```python
from build123d import *

# Parameters (mm, degrees)
SKETCH1_R           = 1.25
BOSS_EXTRUDE1_DEPTH = 3
SKETCH8_R           = 2.45
SKETCH8_R_2         = 1.85
CUT_EXTRUDE3_DEPTH  = 0.8
CHAMFER4_SIZE       = 0.3
SKETCH9_R           = 3.1
CUT_EXTRUDE4_DEPTH  = 20.810156141
BOSS_EXTRUDE2_DEPTH = 14
CUT_EXTRUDE5_REACH  = 27.931
SKETCH11_W          = 1.3
SKETCH11_H          = 2.4
FILLET1_SIZE        = 0.7
FILLET1_SIZE_2      = 1.8
CUT_EXTRUDE6_REACH  = 26.043


# Some blends are built 0.0001 mm under size
with BuildPart() as part:
    # Sketch1 → Boss-Extrude1 (new body)
    with BuildSketch(Plane(origin=(0, 0, 0), x_dir=(1, 0, 0), z_dir=(0, 1, 0))):
        with BuildLine():
            ThreePointArc((4.470296705, 10.516185401), (0, 14.5), (-4.470296705, 10.516185401))
            ThreePointArc((-4.470296705, 10.516185401), (-6.673163323, 3.852752641), (-11.342432061, -1.386702192))
            ThreePointArc((-11.342432061, -1.386702192), (-12.557368355, -7.25), (-6.872135356, -9.12948321))
            ThreePointArc((-6.872135356, -9.12948321), (0, -7.705505282), (6.872135356, -9.12948321))
            ThreePointArc((6.872135356, -9.12948321), (12.557368355, -7.25), (11.342432061, -1.386702192))
            ThreePointArc((11.342432061, -1.386702192), (6.673163323, 3.852752641), (4.470296705, 10.516185401))
        make_face()
        with Locations(Location((0, 10, 0), (0, 0, 270))):
            Circle(SKETCH1_R, mode=Mode.SUBTRACT)
        with Locations(Location((-8.660254038, -5, 0), (0, 0, 270))):
            Circle(SKETCH1_R, mode=Mode.SUBTRACT)
        with Locations(Location((8.660254038, -5, 0), (0, 0, 270))):
            Circle(SKETCH1_R, mode=Mode.SUBTRACT)
    extrude(amount=BOSS_EXTRUDE1_DEPTH)

    # Sketch8 → Cut-Extrude3 (cut)
    # profile 1 of 3: a face of its own
    with BuildSketch(Plane.XZ):
        with Locations(Location((8.660254038, 5, 0), (0, 0, 270))):
            Circle(SKETCH8_R)
        with Locations(Location((8.660254038, 5, 0), (0, 0, 270))):
            Circle(SKETCH8_R_2, mode=Mode.SUBTRACT)
    # profile 2 of 3: a face of its own
    with BuildSketch(Plane.XZ):
        with Locations(Location((-8.660254038, 5, 0), (0, 0, 270))):
            Circle(SKETCH8_R)
        with Locations(Location((-8.660254038, 5, 0), (0, 0, 270))):
            Circle(SKETCH8_R_2, mode=Mode.SUBTRACT)
    # profile 3 of 3: a face of its own
    with BuildSketch(Plane.XZ):
        with Locations(Location((0, -10, 0), (0, 0, 270))):
            Circle(SKETCH8_R)
        with Locations(Location((0, -10, 0), (0, 0, 270))):
            Circle(SKETCH8_R_2, mode=Mode.SUBTRACT)
    extrude(amount=-CUT_EXTRUDE3_DEPTH, mode=Mode.SUBTRACT)

    # Chamfer4
    chamfer4_edges = [part.edges().sort_by_distance(p)[0] for p in [
        (8.660254038, 0.8, 7.45),
        (8.660254038, 0.8, 6.85),
        (-8.660254038, 0.8, 7.45),
        (-8.660254038, 0.8, 6.85),
        (0, 0.8, -7.55),
        (0, 0.8, -8.15),
        (0, 0, -7.55),
    ]]
    chamfer(chamfer4_edges, length=CHAMFER4_SIZE - 0.0001)  # a hair under: the kernel refuses the full size

    # Sketch9 → Cut-Extrude4 (cut, through all)
    with BuildSketch(Plane(origin=(0, 3, 0), x_dir=(1, 0, 0), z_dir=(0, 1, 0))):
        with Locations(Location((0, 0, 0), (0, 0, 270))):
            Circle(SKETCH9_R)
    extrude(amount=-CUT_EXTRUDE4_DEPTH, mode=Mode.SUBTRACT)

    # Sketch10 → Boss-Extrude2 (add)
    with BuildSketch(Plane(origin=(0, 3, 0), x_dir=(1, 0, 0), z_dir=(0, 1, 0))):
        with BuildLine():
            ThreePointArc((-1.25, 7.603440777), (-7.705505282, 0), (-1.25, -7.603440777))
            Line((-1.25, -7.603440777), (-1.25, -5.458708638))
            ThreePointArc((-1.25, -5.458708638), (-5.6, 0), (-1.25, 5.458708638))
            Line((-1.25, 5.458708638), (-1.25, 7.603440777))
        make_face()
        with BuildLine():
            Line((1.25, -5.458708638), (1.25, -7.603440777))
            ThreePointArc((1.25, -7.603440777), (5.873954939, -4.987129939), (7.705505282, 0))
            ThreePointArc((7.705505282, 0), (5.873954939, 4.987129939), (1.25, 7.603440777))
            Line((1.25, 7.603440777), (1.25, 5.458708638))
            ThreePointArc((1.25, 5.458708638), (4.379497688, 3.489985673), (5.6, 0))
            ThreePointArc((5.6, 0), (4.379497688, -3.489985673), (1.25, -5.458708638))
        make_face()
    extrude(amount=BOSS_EXTRUDE2_DEPTH)

    # Sketch11 → Cut-Extrude5 (cut, up to next)
    with BuildSketch(Plane.XZ, mode=Mode.PRIVATE) as cut_extrude5_sk1:
        Polygon((13.271598839, 8.412916512), (11.19313787, 7.212916512), (11.84313787, 6.087083488), (13.921598839, 7.287083488), align=None)
    cut_extrude5_tool1 = extrude(cut_extrude5_sk1.sketch, amount=-CUT_EXTRUDE5_REACH, mode=Mode.PRIVATE) & part.part
    # Sketch11 → Cut-Extrude5 (cut, up to next)
    with BuildSketch(Plane.XZ, mode=Mode.PRIVATE) as cut_extrude5_sk2:
        Polygon((-13.921598839, 7.287083488), (-11.84313787, 6.087083488), (-11.19313787, 7.212916512), (-13.271598839, 8.412916512), align=None)
    cut_extrude5_tool2 = extrude(cut_extrude5_sk2.sketch, amount=-CUT_EXTRUDE5_REACH, mode=Mode.PRIVATE) & part.part
    # Sketch11 → Cut-Extrude5 (cut, up to next)
    with BuildSketch(Plane.XZ, mode=Mode.PRIVATE) as cut_extrude5_sk3:
        with Locations((0, -14.5)):
            Rectangle(SKETCH11_W, SKETCH11_H)
    cut_extrude5_tool3 = extrude(cut_extrude5_sk3.sketch, amount=-CUT_EXTRUDE5_REACH, mode=Mode.PRIVATE) & part.part
    add(cut_extrude5_tool1.solids().sort_by_distance((12.557368, 0, 7.25))[0], mode=Mode.SUBTRACT)
    add(cut_extrude5_tool2.solids().sort_by_distance((-12.557368, 0, 7.25))[0], mode=Mode.SUBTRACT)
    add(cut_extrude5_tool3.solids().sort_by_distance((0, 0, -14.5))[0], mode=Mode.SUBTRACT)

    # Fillet1
    # an asymmetric fillet: 1.8, 0.7 mm, written as the material it adds along each edge
    with BuildSketch(Plane(origin=(0, 3, 0), x_dir=(0.5475293805867771, 0, 0.8367864586585159), z_dir=(0.8367864586585159, 0, -0.5475293805867771))) as fillet1_piece_1_section:
        with BuildLine():
            Bezier((5.6 - FILLET1_SIZE, 0), (5.6, 0), (5.6, -FILLET1_SIZE_2), weights=[1, 0.707106781, 1])
            Line((5.6, -FILLET1_SIZE_2), (5.6, 0))
            Line((5.6, 0), (5.6 - FILLET1_SIZE, 0))
        make_face()
    fillet1_piece_1 = revolve(axis=Axis((0, 3, 0), (0, -1, 0)), revolution_arc=246.395365409, mode=Mode.PRIVATE)
    fillet1_piece_1 = split(fillet1_piece_1, bisect_by=Plane(origin=(1.25, 3.4101004, 4.981961309), z_dir=(1, 0, 0)), keep=Keep.TOP, mode=Mode.PRIVATE)
    add(fillet1_piece_1)
    with BuildSketch(Plane(origin=(0, 3, 0), x_dir=(0.5475293805867771, 0, 0.8367864586585159), z_dir=(0.8367864586585159, 0, -0.5475293805867771))) as fillet1_piece_2_section:
        with BuildLine():
            Bezier((5.6 - FILLET1_SIZE, 0), (5.6, 0), (5.6, -FILLET1_SIZE_2), weights=[1, 0.707106781, 1])
            Line((5.6, -FILLET1_SIZE_2), (5.6, 0))
            Line((5.6, 0), (5.6 - FILLET1_SIZE, 0))
        make_face()
    fillet1_piece_2 = revolve(axis=Axis((0, 3, 0), (0, -1, 0)), revolution_arc=246.395365409, mode=Mode.PRIVATE)
    fillet1_piece_2 = split(fillet1_piece_2, bisect_by=Plane(origin=(-1.25, 3.521482182, 0), z_dir=(-1, 0, 0)), keep=Keep.TOP, mode=Mode.PRIVATE)
    add(fillet1_piece_2)
    with BuildSketch(Plane(origin=(0, 3, 0), x_dir=(-0.5475293805867888, 0, -0.8367864586585083), z_dir=(-0.8367864586585083, 0, 0.5475293805867888))) as fillet1_piece_3_section:
        with BuildLine():
            Bezier((5.6 - FILLET1_SIZE, 0), (5.6, 0), (5.6, -FILLET1_SIZE_2), weights=[1, 0.707106781, 1])
            Line((5.6, -FILLET1_SIZE_2), (5.6, 0))
            Line((5.6, 0), (5.6 - FILLET1_SIZE, 0))
        make_face()
    fillet1_piece_3 = revolve(axis=Axis((0, 3, 0), (0, -1, 0)), revolution_arc=246.395365409, mode=Mode.PRIVATE)
    fillet1_piece_3 = split(fillet1_piece_3, bisect_by=Plane(origin=(-1.25, 3.4101004, -4.981961309), z_dir=(-1, 0, 0)), keep=Keep.TOP, mode=Mode.PRIVATE)
    add(fillet1_piece_3)
    with BuildSketch(Plane(origin=(0, 3, 0), x_dir=(-0.5475293805867888, 0, -0.8367864586585083), z_dir=(-0.8367864586585083, 0, 0.5475293805867888))) as fillet1_piece_4_section:
        with BuildLine():
            Bezier((5.6 - FILLET1_SIZE, 0), (5.6, 0), (5.6, -FILLET1_SIZE_2), weights=[1, 0.707106781, 1])
            Line((5.6, -FILLET1_SIZE_2), (5.6, 0))
            Line((5.6, 0), (5.6 - FILLET1_SIZE, 0))
        make_face()
    fillet1_piece_4 = revolve(axis=Axis((0, 3, 0), (0, -1, 0)), revolution_arc=246.395365409, mode=Mode.PRIVATE)
    fillet1_piece_4 = split(fillet1_piece_4, bisect_by=Plane(origin=(1.25, 3.521482182, 0), z_dir=(1, 0, 0)), keep=Keep.TOP, mode=Mode.PRIVATE)
    add(fillet1_piece_4)

    # Sketch13 → Cut-Extrude6 (cut, up to next)
    with BuildSketch(Plane(origin=(0, 3, 0), x_dir=(1, 0, 0), z_dir=(0, 1, 0)), mode=Mode.PRIVATE) as cut_extrude6_sk1:
        with BuildLine():
            Line((-1.2, 3.520347662), (-1.2, 2.858321186))
            ThreePointArc((-1.2, 2.858321186), (1.71610023, 2.581666129), (3.1, 0))
            ThreePointArc((3.1, 0), (3.079772307, -0.353556981), (3.019353201, -0.7025))
            ThreePointArc((3.019353201, -0.7025), (3.1918175, -0.112209971), (3.25, 0.5))
            ThreePointArc((3.25, 0.5), (1.825171225, 3.189098362), (-1.2, 3.520347662))
        make_face()
    cut_extrude6_tool1 = extrude(cut_extrude6_sk1.sketch, amount=-CUT_EXTRUDE6_REACH, mode=Mode.PRIVATE) & part.part
    add(cut_extrude6_tool1.solids().sort_by_distance((1.789819, 3, -3.137012))[0], mode=Mode.SUBTRACT)

    # Fillet2
    # an asymmetric fillet: 0.5, 0.4 mm, written as the material it adds along each edge
    with BuildSketch(Plane(origin=(-1.2, 3, -3.520347662), x_dir=(0.9513626370568626, 0, -0.3080732588398615), z_dir=(0, -1, 0))) as fillet2_piece_1:
        with BuildLine():
            Bezier((0.422293635, 0), (0.008719291, -0.026926088), (-0.079374984, 0.245118303), weights=[1, 0.789181232, 1])
            Line((-0.079374984, 0.245118303), (0, 0))
            ThreePointArc((0, 0), (0.211146817, -0.006866173), (0.422293635, 0))
        make_face()
    extrude(amount=3)


solid = part.part
```
Geometry: final body of the model. Coordinates: model frame, mm. A direction names the side the tool comes from. Round coordinates to 2 decimals unless told otherwise and drop trailing zeros. Use CSV: the item, a comma, the result in double quotes. Start each with the question number.
Q1. Line query: L1, parallel to X at y = 1.55, z = 5; L2, parallel to X at y = 2, z = 4; L3, parallel to Y at x = -11.25, z = 7.5. Output: solid intervals per line, ascending.
Q2. Reachability of faces 5 (the face through (6.487, 0.247, 3.869)), 6 (the face through (-12.978, 1.479, 3.731)), 7 (the face through (-0.65, 1, -14)), 8 (the face through (12.335, 1.479, 6.371)) from +Z, -Z, +X, -X, +Y, -Y: full face, straight path, thin tool, end or side. Return the list, or none.
Q3. First-contact query: pin 1 Ø4 at (x, y) = (-4, 12.5) entering from -Z; pin 2 Ø4.5 at (x, z) = (0, -10) entering from -Y; pin 3 Ø2 at (y, z) = (12, 4.5) entering from +X; pin 4 Ø1.4 at (y, z) = (7, 6.5) entering from +X. Flat tips, straight axial feed; report the tip coordinate or a pass-through.
Q4. Section B-B (x = 0). Give the number of separate pieces and of enclosed holes in the cut face, plus the area to 3 significant figures.
Q5. Pull-direction query (X, two-part tool) for faces 1 (the face through (0, 0, -4)), 2 (the face through (-5.6, 10.8, 0.1)), 3 (the face through (0, 1, -13.3)), 4 (the face through (-6.624, 1.479, -3.939)); classes: pulls with the +X half, pulls with the -X half, needs draft (parallel to the pull), parting line crosses it, or undercut.
Result sheet:
1,L1,"-13.16 to -9.91, -7.41 to 7.41, 9.91 to 13.16"
1,L2,"-13.05 to -9.41, -7.91 to 7.91, 9.41 to 13.05"
1,L3,"0 to 3"
2,face 5,"-Y"
2,face 6,"-X, +Y, -Y"
2,face 7,"-Z, +Y, -Y"
2,face 8,"+Y, -Y"
3,pin 1,"z = -7.44"
3,pin 2,"y = 0"
3,pin 3,"x = 6.86"
3,pin 4,"x = 5.07"
4,separate pieces,"3"
4,enclosed holes,"0"
4,area,"34.1 mm²"
5,face 1,"needs draft"
5,face 2,"undercut"
5,face 3,"undercut"
5,face 4,"pulls with the -X half"
